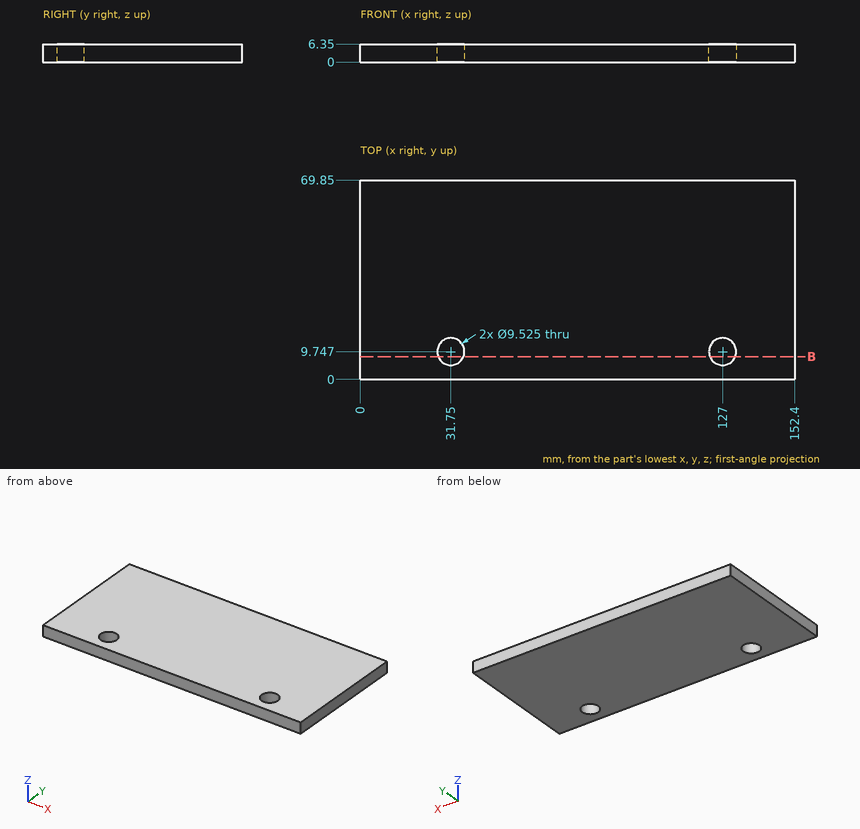
Can you work these out from the drawing? Everything is in mm from the part's minimum corner. Round coordinates to 2 decimals unless told otherwise and drop trailing zeros. Order: outer loops, then holes, each group sorted by start corner. A loop starts at its lowest first (then second) coordinate and runs counter-clockwise, first axis right, second up. Notation, with made-up numbers: (-6.5, 45.5) - (43.5, 45.5) arc R21 cw to (43.5, 61.5) - close; hole circle Ø9 at (-2.5, 29.25). An arc over 180 degrees is marked (long way). Answer in a Markdown table with one row per item.
(1) For P1, Ø3, axis at x = 100.5, y = 38.5, coming from the -Z side; P2, Ø5.5, axis at x = 31.75, y = 9.75, coming from the +Z side, each with a flat end and sliding along its axis, tell me the tip position at first contact or that it passes through.
From the geometry:
| item | result |
|---|---|
| P1 | stops at z = 0 |
| P2 | passes through |
(2) Please list where these lines run through material, in increasing order: L1, parallel to X at y = 8, z = 6.25; L2, parallel to X at y = 12, z = 1.75 (1 decimal); L3, parallel to Y at x = 33, z = 5. Write a range as from..to.
From the geometry:
| item | result |
|---|---|
| L1 | x = 0..27.32, 36.18..122.57, 131.43..152.4 |
| L2 | x = 0..27.6, 35.9..122.8, 131.2..152.4 |
| L3 | y = 0..5.15, 14.34..69.85 |
(3) Suppose I cut it at B-B, the plane y = 8. Please give me the cut outline in (x, z).
From the geometry:
| item | result |
|---|---|
| outline | (0, 0) - (27.32, 0) - (27.32, 6.35) - (0, 6.35) - close; (36.18, 0) - (122.57, 0) - (122.57, 6.35) - (36.18, 6.35) - close; (131.43, 0) - (152.4, 0) - (152.4, 6.35) - (131.43, 6.35) - close |
